```python
from build123d import *

# Parameters (mm, degrees)
BOSS_EXTRUDE1_DEPTH = 6.5


with BuildPart() as part:
    # Sketch1 → Boss-Extrude1 (new, symmetric)
    with BuildSketch(Plane(origin=(0, 0, 0), x_dir=(1, 0, 0), z_dir=(0, 1, 0))):
        with BuildLine():
            ThreePointArc((1.625, 0), (1.381801361, 0.855131569), (0.725, 1.454303957))
            Line((0.725, 1.454303957), (0.725, -1.454303957))
            ThreePointArc((0.725, -1.454303957), (1.381801361, -0.855131569), (1.625, 0))
        make_face()
        with BuildLine():
            ThreePointArc((0.725, 1.454303957), (0, 1.625), (-0.725, 1.454303957))
            Line((-0.725, 1.454303957), (-0.725, -1.454303957))
            ThreePointArc((-0.725, -1.454303957), (0, -1.625), (0.725, -1.454303957))
            Line((0.725, -1.454303957), (0.725, 1.454303957))
        make_face()
        with BuildLine():
            Line((-0.725, -1.454303957), (-0.725, 1.454303957))
            ThreePointArc((-0.725, 1.454303957), (-1.625, 0), (-0.725, -1.454303957))
        make_face()
        with BuildLine():
            Line((0.725, 2.975), (-0.725, 2.975))
            Line((-0.725, 2.975), (-0.725, 1.454303957))
            ThreePointArc((-0.725, 1.454303957), (0, 1.625), (0.725, 1.454303957))
            Line((0.725, 1.454303957), (0.725, 2.975))
        make_face()
        with BuildLine():
            ThreePointArc((0.725, -1.454303957), (0, -1.625), (-0.725, -1.454303957))
            Line((-0.725, -1.454303957), (-0.725, -2.975))
            Line((-0.725, -2.975), (0.725, -2.975))
            Line((0.725, -2.975), (0.725, -1.454303957))
        make_face()
    extrude(amount=BOSS_EXTRUDE1_DEPTH, both=True)


solid = part.part
```
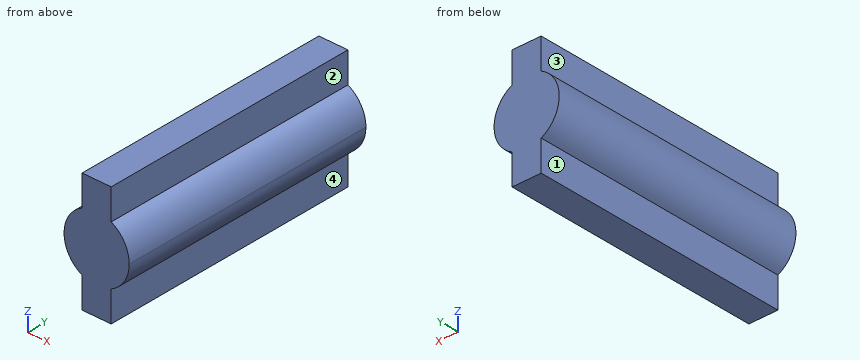
Verification items for the finished model (mm, model axes). Face numbers are marked on the shaded views. A direction names the side the tool comes from. Round coordinates to 2 decimals unless told otherwise and drop trailing zeros. Write each loop counter-clockwise with the first axis right and the second up, starting at its lowest first coordinate (ties: lowest second). Pieces come first, ordered by that corner, then holes.
1. Gauge pin test, flat ends, axial feed: P1, Ø1.2, axis at y = 2, z = -2, coming from the +X side (3 decimals); P2, Ø0.8, axis at y = 1.5, z = 2, coming from the +X side (3 decimals); P3, Ø1.2, axis at y = 1.5, z = 2, coming from the -X side (3 decimals). Record the tip position at first contact, or that the pin passes through.
2. Section check B-B on x = -1.2. Enter the section's corners in (y, z).
3. Section check C-C on z = 1.65. Enter the section's corners in (x, y) (3 decimals), plus the area to 4 significant figures.
4. Section check A-A on y = 3.25. Enter the section's corners in (x, z) (3 decimals).
5. Access from +Z, -Z, +X, -X, +Y, -Y to the whole of each face (thin tool, end or side, straight path). Record for the marked faces 1, 2, 3 and 4.
6. Scan lines: L1, parallel to X at y = 0.75, z = -2.6 (3 decimals); L2, parallel to Z at x = 1.3, y = 4 (3 decimals); L3, parallel to Z at x = 1.4, y = -2.75 (3 decimals). Record each from-to range of solid material in increasing order.
Answer:
1. P1: stops at x = 0.825
1. P2: stops at x = 0.725
1. P3: stops at x = -0.825
2. outline: (-6.5, -1.1) - (6.5, -1.1) - (6.5, 1.1) - (-6.5, 1.1) - close
3. outline: (-0.725, -6.5) - (0.725, -6.5) - (0.725, 6.5) - (-0.725, 6.5) - close
3. area: 18.85 mm2
4. outline: (-0.725, -2.975) - (0.725, -2.975) - (0.725, -1.454) arc R1.625 ccw to (0.725, 1.454) - (0.725, 2.975) - (-0.725, 2.975) - (-0.725, 1.454) arc R1.625 ccw to (-0.725, -1.454) - close
5. face 1: -Z, -X, +Y, -Y
5. face 2: +Z, +X, +Y, -Y
5. face 3: +Z, -X, +Y, -Y
5. face 4: -Z, +X, +Y, -Y
6. L1: x = -0.725 to 0.725
6. L2: z = -0.975 to 0.975
6. L3: z = -0.825 to 0.825
